Work out the finished part from the listing and answer in its coordinate system (mm). Round coordinates to 2 decimals unless told otherwise and drop trailing zeros. Order: outer loops, then holes, each group sorted by start corner. A loop starts at its lowest first (then second) coordinate and runs counter-clockwise, first axis right, second up. Notation, with made-up numbers: (4.25, -30.5) - (46.25, -30.5) arc R14 ccw to (46.25, -5.5) - close; hole circle Ø4 at (19, -5). An arc over 180 degrees is marked (long way). Use CSV: the item, a comma, the result in double quotes.
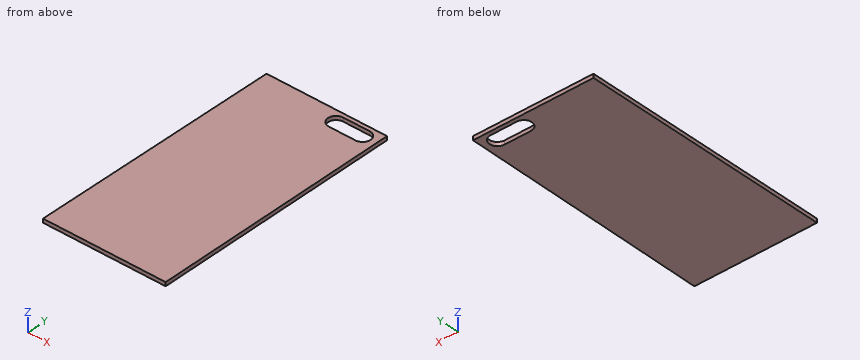
from build123d import *

# Parameters (mm, degrees)
F1_DEPTH = 1.9431
F3_DEPTH = 25.4


with BuildPart() as f1:
    # F0 (on Top) → F1 (new body)
    with BuildSketch(Plane.XY):
        Polygon((27.7205, 0), (-32.982886, 0), (-34.080576, -125.857264), (27.7205, -125.857264), align=None)
    extrude(amount=F1_DEPTH)

    # F2 (on face) → F3 (cut)
    with BuildSketch(Plane.XY.offset(1.9431)):
        with BuildLine():
            Line((7.332415, -4.307757), (7.332415, -1.955202))
            ThreePointArc((7.332415, -1.955202), (3.332973, -5.954644), (7.332415, -9.954086))
            Line((7.332415, -9.954086), (7.332415, -4.307757))
        make_face()
        Polygon((14.004417, -4.307757), (14.004417, -1.955202), (7.332415, -1.955202), (7.332415, -4.307757), (7.332415, -9.954086), (14.004417, -9.954086), align=None)
        with BuildLine():
            Line((20.676419, -1.955202), (20.676419, -4.307757))
            Line((20.676419, -4.307757), (20.676419, -9.954086))
            ThreePointArc((20.676419, -9.954086), (24.675861, -5.954644), (20.676419, -1.955202))
        make_face()
        Polygon((20.676419, -9.954086), (20.676419, -4.307757), (20.676419, -1.955202), (14.004417, -1.955202), (14.004417, -4.307757), (14.004417, -9.954086), (14.634087, -9.954086), align=None)
    extrude(amount=-F3_DEPTH, mode=Mode.SUBTRACT)


solid = f1.part
(1) Find section A-A (z = 0.8). Determine the outline of the cut face in (x, y), and give its area (3 significant figures).
Findings below:
outline,"(-34.08, -125.86) - (27.72, -125.86) - (27.72, 0) - (-32.98, 0) - close; hole (7.33, -9.95) - (20.68, -9.95) arc R4 ccw to (20.68, -1.96) - (7.33, -1.96) arc R4 ccw to start"
area,"7,550 mm²"
(2) Find section C-C (y = -18.5). Determine the outline of the cut face in (x, z).
Findings below:
outline,"(-33.14, 0) - (27.72, 0) - (27.72, 1.94) - (-33.14, 1.94) - close"
(3) Find section B-B (x = 12). Determine the outline of the cut face in (y, z).
Findings below:
outline,"(-125.86, 0) - (-9.95, 0) - (-9.95, 1.94) - (-125.86, 1.94) - close; (-1.96, 0) - (0, 0) - (0, 1.94) - (-1.96, 1.94) - close"
(4) Find the intervals of material crossed by L1, parallel to Y at x = 8.5, z = 0.15; L2, parallel to Y at x = 7, z = 0.8; L3, parallel to X at y = -108, z = 0.3, in increasing order. Write a range as from..to.
Findings below:
L1,"y = -125.86..-9.95, -1.96..0"
L2,"y = -125.86..-9.94, -1.97..0"
L3,"x = -33.92..27.72"
